Here's how the part is built. I have some questions about the finished solid (model axes, mm). A direction names the side the tool comes from. Round coordinates to 2 decimals unless told otherwise and drop trailing zeros. Loops run counter-clockwise (first coordinate to the right, second up) from the corner with the lowest first, then second, coordinate; pieces in that order, holes last. Notation, with made-up numbers: M 34.25,-9 L 59.25,-9 A11 cw 59.25,3 Z; hole C -16,83 d2. An arc over 180 degrees is marked long. Answer as a JSON object with one key per item and string values.
from build123d import *

# Parameters (mm, degrees)
SKETCH1_W           = 406.4
SKETCH1_H           = 25.4
SKETCH1_W_2         = 76.2
SKETCH1_H_2         = 38.1
BOSS_EXTRUDE1_DEPTH = 6.35
SKETCH3_R           = 2.794
CUT_EXTRUDE2_DEPTH  = 6.35
FILLET1_R           = 12.7
SKETCH4_R           = 2.794
CUT_EXTRUDE3_DEPTH  = 19.05
SKETCH5_R           = 5.08
CUT_EXTRUDE4_DEPTH  = 3.175
SKETCH6_W           = 88.9
SKETCH6_H           = 25.4
CUT_EXTRUDE5_DEPTH  = 6.35


with BuildPart() as part:
    # Sketch1 → Boss-Extrude1 (new body)
    with BuildSketch(Plane(origin=(0, 0, 0), x_dir=(1, 0, 0), z_dir=(0, 1, 0))):
        with Locations((203.2, 12.7)):
            Rectangle(SKETCH1_W, SKETCH1_H)
        with Locations((203.2, 44.45)):
            Rectangle(SKETCH1_W_2, SKETCH1_H_2)
    extrude(amount=BOSS_EXTRUDE1_DEPTH)

    # Sketch3 → Cut-Extrude2 (cut)
    with BuildSketch(Plane(origin=(0, 6.35, 0), x_dir=(1, 0, 0), z_dir=(0, 1, 0))):
        with Locations(Location((222.25, 50.8, 0), (0, 0, 270))):
            Circle(SKETCH3_R)
        with Locations(Location((184.15, 50.8, 0), (0, 0, 270))):
            Circle(SKETCH3_R)
    extrude(amount=-CUT_EXTRUDE2_DEPTH, mode=Mode.SUBTRACT)

    # Fillet1
    fillet1_edges = [part.edges().sort_by_distance(p)[0] for p in [
        (406.4, 3.175, 0),
        (406.4, 3.175, -25.4),
        (0, 3.175, 0),
        (0, 3.175, -25.4),
        (165.1, 3.175, -25.4),
        (241.3, 3.175, -25.4),
        (241.3, 3.175, -63.5),
        (165.1, 3.175, -63.5),
    ]]
    fillet(fillet1_edges, radius=FILLET1_R - 0.0001)  # a hair under: the kernel refuses the full size

    # Sketch4 → Cut-Extrude3 (cut)
    with BuildSketch(Plane(origin=(0, 6.35, 0), x_dir=(1, 0, 0), z_dir=(0, 1, 0))):
        with Locations(Location((279.4, 12.7, 0), (0, 0, 270))):
            Circle(SKETCH4_R)
        with Locations(Location((304.8, 12.7, 0), (0, 0, 270))):
            Circle(SKETCH4_R)
        with Locations(Location((127, 12.7, 0), (0, 0, 270))):
            Circle(SKETCH4_R)
        with Locations(Location((101.6, 12.7, 0), (0, 0, 270))):
            Circle(SKETCH4_R)
    extrude(amount=-CUT_EXTRUDE3_DEPTH, mode=Mode.SUBTRACT)

    # Sketch5 → Cut-Extrude4 (cut)
    with BuildSketch(Plane(origin=(0, 6.35, 0), x_dir=(1, 0, 0), z_dir=(0, 1, 0))):
        with Locations(Location((101.6, 12.7, 0), (0, 0, 270))):
            Circle(SKETCH5_R)
        with Locations(Location((127, 12.7, 0), (0, 0, 270))):
            Circle(SKETCH5_R)
        with Locations(Location((279.4, 12.7, 0), (0, 0, 270))):
            Circle(SKETCH5_R)
        with Locations(Location((304.8, 12.7, 0), (0, 0, 270))):
            Circle(SKETCH5_R)
    extrude(amount=-CUT_EXTRUDE4_DEPTH, mode=Mode.SUBTRACT)

    # Sketch6 → Cut-Extrude5 (cut)
    with BuildSketch(Plane(origin=(0, 6.35, 0), x_dir=(1, 0, 0), z_dir=(0, 1, 0))):
        with Locations((44.45, 12.7)):
            Rectangle(SKETCH6_W, SKETCH6_H)
        with Locations((361.95, 12.7)):
            Rectangle(SKETCH6_W, SKETCH6_H)
    extrude(amount=-CUT_EXTRUDE5_DEPTH, mode=Mode.SUBTRACT)


solid = part.part
Item 1: I want a section at D-D on z = -44.5. List the corners of the cut face in (x, y) for me, plus the area to 3 significant figures.
Solution:
{"outline": "M 165.1,0 L 241.3,0 L 241.3,6.35 L 165.1,6.35 Z", "area": "484 mm2"}
Item 2: We'd pull the mould along Z, two halves only. Please class faces 6 (the face through (165.1, 3, -44)), 7 (the face through (302.6, 3.175, -10.5)), 8 (the face through (203, 3, -63.5)): +Z half, -Z half, draft (parallel to the pull), parting line (faces both ways), or undercut.
Solution:
{"face 6": "draft", "face 7": "undercut", "face 8": "-Z half"}
Item 3: For faces 1 (the face through (186.92, 3.22, -51.16)), 2 (the face through (122.04, 4.78, -13.8)), 3 (the face through (202, 3, 0)), 4 (the face through (285, 3, -25.4)), 5 (the face through (120, 3, -25.4)), which set-ups out of +Z, -Z, +X, -X, +Y, -Y let a thin tool reach every point of the face, with its end or its side?
Solution:
{"face 1": "+Y, -Y", "face 2": "+Y", "face 3": "+Z, +X, -X, +Y, -Y", "face 4": "-Z, +X, +Y, -Y", "face 5": "-Z, -X, +Y, -Y"}
Item 4: I want a section at C-C on x = 184.15. List the corners of the cut face in (y, z) for me, plus the area to 3 significant figures.
Solution:
{"outline": "M 0,-63.5 L 6.35,-63.5 L 6.35,-53.59 L 0,-53.59 Z; M 0,-48.01 L 6.35,-48.01 L 6.35,0 L 0,0 Z", "area": "368 mm2"}
Item 5: If I drill on L1, parallel to X at y = 0.9, z = -12.7; L2, parallel to X at y = 3.9, z = -12.7; L3, parallel to Z at x = 222.25, y = 2, over which ranges is the centre line in solid material (lowest first)? Write a range as from..to.
Solution:
{"L1": "x = 88.9..98.81, 104.39..124.21, 129.79..276.61, 282.19..302.01, 307.59..317.5", "L2": "x = 88.9..96.52, 106.68..121.92, 132.08..274.32, 284.48..299.72, 309.88..317.5", "L3": "z = -63.5..-53.59, -48.01..0"}
Item 6: For P1, Ø3.5, axis at x = 279.4, z = -12.7, coming from the +Y side; P2, Ø3, axis at x = 99.5, z = -11, coming from the +Y side (3 decimals); P3, Ø1.9, axis at y = 2.5, z = -44.5, coming from the +X side; P4, Ø1.9, axis at x = 132, y = 2, coming from the -Z side, each with a flat end and sliding along its axis, tell me the tip position at first contact or that it passes through.
Solution:
{"P1": "passes through", "P2": "stops at y = 3.175", "P3": "stops at x = 241.3", "P4": "stops at z = -25.4"}
Item 7: I want a section at B-B on z = -12.7. Count the separate pieces of the cut face and the enclosed holes in it, plus the area to 3 significant figures.
Solution:
{"separate pieces": "5", "enclosed holes": "0", "area": "1,250 mm2"}
Item 8: I want a section at A-A on x = 279.4. List the corners of the cut face in (y, z) for me (3 decimals).
Solution:
{"outline": "M 0,-25.4 L 6.35,-25.4 L 6.35,-17.78 L 3.175,-17.78 L 3.175,-15.494 L 0,-15.494 Z; M 0,-9.906 L 3.175,-9.906 L 3.175,-7.62 L 6.35,-7.62 L 6.35,0 L 0,0 Z"}
